```python
from build123d import *

# Parameters (mm, degrees)
F1_DEPTH = 2


with BuildPart() as f1:
    # F0 (on Right) → F1 (new body)
    with BuildSketch(Plane.YZ):
        with BuildLine():
            ThreePointArc((-3.6381939636, 9.3146950934), (8.257782379, -5.639949484), (-10, 0))
            ThreePointArc((-10, 0), (-10.2934540428, 2.639788856), (-10.791214382, 5.2487800641))
            add(Edge.make_bspline(
                [(-10.791214382, 5.2487800641), (-10.8154983711, 6.0263408015), (-10.8550299677, 7.5670980598), (-12.3278240582, 9.3781898524), (-14.520874836, 10.293629199), (-15.7277697161, 10.5687391244), (-16.2077791764, 10.6652913886)],
                knots=[0, 0, 0, 0, 0.1757337799, 0.3486956058, 0.5366450397, 0.6536048932, 0.6536048932, 0.6536048932, 0.6536048932], degree=3))
            Line((-16.2077791764, 10.6652913886), (-18.6808016236, 10.6652913886))
            add(Edge.make_bspline(
                [(-18.6808016236, 10.6652913886), (-18.8148572024, 10.3772405868), (-18.7289432635, 9.8841331089), (-18.6430066824, 9.3909176067)],
                knots=[0.8827630608, 0.8827630608, 0.8827630608, 0.8827630608, 1, 1, 1, 1], degree=3))
            add(Edge.make_bspline(
                [(-11.9811552234, 0.6722495916), (-11.9564777557, 1.6261020361), (-11.9298565867, 3.7922413277), (-12.3964002274, 7.4877698942), (-15.2123230374, 8.8798414319), (-17.7170112276, 9.3591077307), (-18.3933537904, 9.3823415089), (-18.6430066824, 9.3909176067)],
                knots=[0.0450488473, 0.0450488473, 0.0450488473, 0.0450488473, 0.2364437545, 0.4744993228, 0.6873004248, 0.8845757201, 1, 1, 1, 1], degree=3))
            add(Edge.make_bspline(
                [(-12, 0), (-11.9934817942, 0.2238701027), (-11.9869635883, 0.4477402053), (-11.9811552234, 0.6722495916)],
                knots=[0, 0, 0, 0, 0.0450488473, 0.0450488473, 0.0450488473, 0.0450488473], degree=3))
            ThreePointArc((-12, 0), (7.0831374558, -9.686545503), (3.6381939636, 11.4351888783))
            Line((3.6381939636, 11.4351888783), (-3.6381939636, 11.4351888783))
            Line((-3.6381939636, 11.4351888783), (-3.6381939636, 9.3146950934))
        make_face()
    extrude(amount=F1_DEPTH)


solid = f1.part
```
The model under review builds one solid part; all positions refer to its coordinate system, in mm. A direction names the side the tool comes from. Round coordinates to 2 decimals unless told otherwise and drop trailing zeros. Order: outer loops, then holes, each group sorted by start corner. A loop starts at its lowest first (then second) coordinate and runs counter-clockwise, first axis right, second up.
Item 1: Machinability: for faces 4 (the flat face through (1, -3.638, 10)), 5 (the flat face through (1, 0, 11.435)), which of the approach directions +Z, -Z, +X, -X, +Y, -Y give a long, thin tool a straight path to every point of the face, cutting with its end or side? Answer none if there is none.
Working result:
face 4: +Z, +X, -X
face 5: +Z, +X, -X, +Y, -Y
Item 2: To check wall thickness, follow probe 1 along Z at (x, y) = (0.9, 0); probe 2 along Y at (x, z) = (1, 0); probe 3 along Z at (x, y) = (0.45, 1). State the ranges of each line that lie inside material, in increasing order.
Working result:
probe 1: z = -12 to -10, 10 to 11.44
probe 2: y = -12 to -10, 10 to 12
probe 3: z = -11.96 to -9.95, 9.95 to 11.44
Item 3: For pin 1 (1 mm diameter, centred on x = 1.5, z = -7.5, fed in from +Y), flat-tipped, find the tip position at first contact; note if it passes through.
Working result:
pin 1: stops at y = 9.75
Item 4: Add section A-A, the plane y = 0. State the section outline as (x, z) points.
Working result:
outline: (0, -12) - (2, -12) - (2, -10) - (0, -10) - close; (0, 10) - (2, 10) - (2, 11.44) - (0, 11.44) - close
Item 5: Draft analysis for pull direction Z (two halves, no side actions). For faces 1 (the flat face through (1, -17, 10.665)), 2 (the flat face through (0, -5, -9)), 3 (the cylindrical face through (0.986, 8.453, -5.343)), state which applies: released by +Z, released by -Z, zero draft, split by the parting line, or undercut.
Working result:
face 1: released by +Z
face 2: zero draft
face 3: undercut
Item 6: Add section B-B, the plane z = -8.5. State the section outline as (x, y) points.
Working result:
outline: (0, -8.47) - (2, -8.47) - (2, -5.27) - (0, -5.27) - close; (0, 5.27) - (2, 5.27) - (2, 8.47) - (0, 8.47) - close
